Drawing for the job (mm, zero at the part's lowest x, y, z). Coordinates: 2 decimals unless noted, no trailing zeros. Order: outer loops, then holes, each group sorted by start corner. A loop starts at its lowest first (then second) coordinate and runs counter-clockwise, first axis right, second up. Notation, with made-up numbers: M 42.5,-13 L 57.5,-13 A13 ccw 57.5,5 Z; hole C 26,-20 d2. An arc over 180 degrees is marked long. Write item = value, one per line. Start each with the question number.
Q1. Pull direction X, two halves, no side cores. Call the marked faces 1, 2 and 3: released by +X, released by -X, zero draft, split by the parting line, or undercut.
Q2. Band-saw the part on D-D on y = 8.5. Write the cut outline in (x, z), plus the area to 3 significant figures.
Q3. Band-saw the part on C-C on x = 85. Write the cut outline in (y, z).
Q4. Band-saw the part on A-A on y = 23.5. Write the cut outline in (x, z).
Q5. Pin check, flat tips, straight feed: P1, Ø16.5, axis at x = 89, y = 9.5, coming from the -Z side; P2, Ø1, axis at x = 131.5, z = 41, coming from the +Y side; P3, Ø5, axis at y = 10, z = 3, coming from the +X side; P4, Ø5, axis at y = 14.5, z = 2.5, coming from the -X side. Stop position of each tip, or through.
Q6. Drill centre lines: probe 1 along X at (y, z) = (25.25, 90); probe 2 along X at (y, z) = (2, 89); probe 3 along Y at (x, z) = (116.5, 134.5). Where is each one in solid material? Low to high.
Q7. Band-saw the part on B-B on z = 90. Write the cut outline in (x, y).
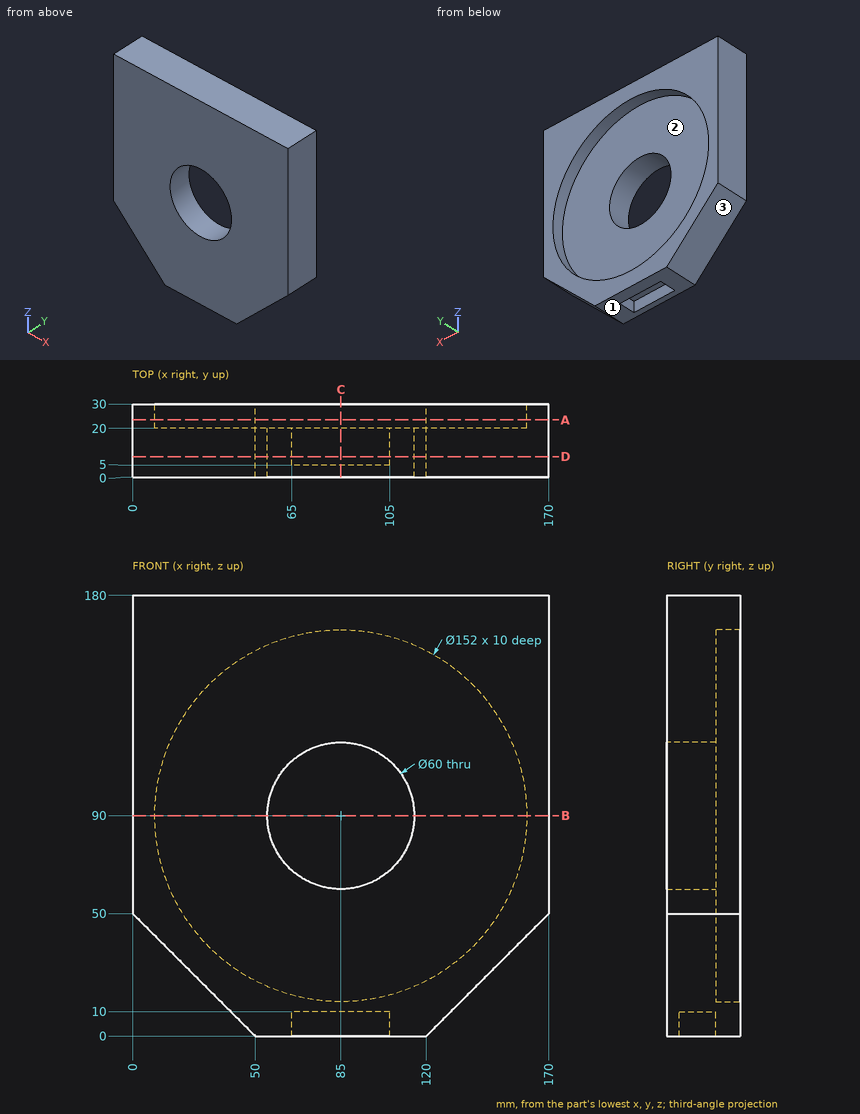
Recorded:
q1.face_1 = zero draft
q1.face_2 = undercut
q1.face_3 = released by -X
q2.outline = M 0,50 L 50,0 L 65,0 L 65,10 L 105,10 L 105,0 L 120,0 L 170,50 L 170,180 L 0,180 Z; hole C 85,90 d60
q2.area = 24,900 mm2
q3.outline = M 0,0 L 5,0 L 5,10 L 20,10 L 20,0 L 30,0 L 30,14 L 20,14 L 20,60 L 0,60 Z; M 0,120 L 20,120 L 20,166 L 30,166 L 30,180 L 0,180 Z
q4.outline = M 0,50 L 50,0 L 120,0 L 170,50 L 170,180 L 0,180 Z; hole C 85,90 d152
q5.P1 = 0
q5.P2 = 20
q5.P3 = 125.5
q5.P4 = 45
q6.probe_1 = 0 to 9, 161 to 170
q6.probe_2 = 0 to 55.02, 114.98 to 170
q6.probe_3 = 0 to 20
q7.outline = M 0,0 L 55,0 L 55,20 L 9,20 L 9,30 L 0,30 Z; M 115,0 L 170,0 L 170,30 L 161,30 L 161,20 L 115,20 Z
